Autodesk Inventor part; units mm, degrees
ref_plane "YZ Plane" through (0, 0, 0) normal (1, 0, 0) x (0, 1, 0)
ref_plane "XZ Plane" through (0, 0, 0) normal (0, 1, 0) x (-1, 0, 0)
ref_plane "XY Plane" through (0, 0, 0) normal (0, 0, 1) x (1, 0, 0)
sketch "Skizze1" plane through (0, 0, 0) normal (0, 0, 1) x (1, 0, 0)
  arc A0 (2.449, 9.6955) -> (2.449, -9.6955) centre (0, 0) ccw
  arc A1 (25.4796, -3.8782) -> (25.4796, 3.8782) centre (24.5, 0) ccw
  line L0 (25.4796, 3.8782) -> (2.449, 9.6955)
  line L1 (25.4796, -3.8782) -> (2.449, -9.6955)
  circle A2 centre (0, 0) radius 3.8
  dimension "d0" = 20
  dimension "d1" = 8
  dimension "d2" = 24.5
  dimension "d40" = 7.6
extrude "Extrusion1" add sketch "Skizze1" along normal blind 3.2
sketch "Skizze2" plane through (0, 0, 0) normal (0, 0, -1) x (-1, 0, 0)
  arc A0 (-25.4796, 3.8782) -> (-25.4796, -3.8782) centre (-24.5, 0) ccw
  circle A1 centre (-24.5, 0) radius 4
  point P0 (0, 0)
  point P1 (-25.4796, 3.8782)
extrude "Extrusion2" add sketch "Skizze2" along normal blind 1.2
sketch "Skizze3" plane through (24.5, 0, -1.2) normal (0, 0, -1) x (-1, 0, 0)
  circle A0 centre (0, 0) radius 4
  point P0 (24.5, 0)
hole "Bohrung1" at (24.5, 0, -1.2) direction (0, 0, 1) diameter 6.2 depth 2
sketch "Skizze4" plane through (0, 0, 0) normal (0, 0, -1) x (-1, 0, 0)
  point P0 (0, 0)
  point P1 (0, -7)
  dimension "d14" = 7
hole "Bohrung2" at (0, -7, 0) direction (0, 0, 1) diameter 2.5 end through all
pattern_circular "Runde Anordnung1" count 4 over 360 about axis through (0, 0, 0) along (0, 0, 1) of "Bohrung2"
chamfer "Fasen4" distance 0.2 angle 45 1 edges at (24.5, -3.1, -1.2)
sketch "Skizze5" plane through (24.5, 0, 0.8) normal (0, 0, -1) x (-1, 0, 0)
  circle A0 centre (0, 0) radius 3.1
  point P0 (24.5, 0)
extrude "Extrusion3" cut sketch "Skizze5" against normal blind 0.5
properties part number "Magnet-arm"
Design review of the part built by this model. Coordinates are the model's own, in mm. A direction names the side the tool comes from. Round coordinates to 2 decimals unless told otherwise and drop trailing zeros. Loops run counter-clockwise (first coordinate to the right, second up) from the corner with the lowest first, then second, coordinate; pieces in that order, holes last. Notation, with made-up numbers: (53.5, -16.75) - (108.5, -16.75) arc R33 ccw to (108.5, 12.25) - close; hole circle Ø10 at (39.25, -19). An arc over 180 degrees is marked (long way). One line per item, written item: value. Start each with the question number.
1) Consider section B-B on z = 2.65. Give the boundary of the cut face in (x, y), then the cut area to 3 significant figures.
2) Draft analysis for pull direction Y (two halves, no side actions). For faces 1 (the flat face through (14.126, -6.746, 1.578)), 2 (the cylindrical face through (21.767, 1.463, 0.166)), 3 (the cylindrical face through (-10, 0, 2)), state which applies: +Y half, -Y half, draft (parallel to the pull), parting line (faces both ways), or undercut.
3) Consider section C-C on y = 0. Give the boundary of the cut face in (x, z), then the cut area to 3 significant figures.
4) To check wall thickness, follow L1, parallel to Z at x = 25.5, y = 1.75; L2, parallel to Y at x = 24.5, z = -0.2; L3, parallel to Z at x = 10, y = 6.75. State the ranges of each line that lie inside material, in increasing order. Write a range as from..to.
5) Consider section A-A on x = 0. Give the boundary of the cut face in (y, z), then the cut area to 3 significant figures.
6) Insertion check: pin 1 Ø2 at (x, z) = (-3.5, 2.5) entering from +Y; pin 2 Ø3 at (x, y) = (-7, 0) entering from -Z; pin 3 Ø1.5 at (x, z) = (23.5, 0.5) entering from +Y. Each pin has a flat end and moves straight along its axis. Give the tip position at first contact, or say it passes through.
7) Consider section D-D on x = 7. Give the boundary of the cut face in (y, z).
8) For faces 4 (the cylindrical face through (8.25, -0.05, 1.62)), 5 (the flat face through (25, 0, 1.3)), list the 3-axis set-ups (+Z, -Z, +X, -X, +Y, -Y) from which the entire face can be reached by the end or side of a thin tool; tool diameter is ignored.
Reported:
1. outline: (2.45, -9.7) - (25.48, -3.88) arc R4 ccw to (25.48, 3.88) - (2.45, 9.7) arc R10 ccw (long way) to start; hole circle Ø2.5 at (-7, 0); hole circle Ø7.6 at (0, 0); hole circle Ø2.5 at (0, -7); hole circle Ø2.5 at (0, 7); hole circle Ø2.5 at (7, 0)
1. area: 471 mm^2
2. face 1: -Y half
2. face 2: undercut
2. face 3: parting line
3. outline: (-10, 0) - (-8.25, 0) - (-8.25, 3.2) - (-10, 3.2) - close; (-5.75, 0) - (-3.8, 0) - (-3.8, 3.2) - (-5.75, 3.2) - close; (3.8, 0) - (5.75, 0) - (5.75, 3.2) - (3.8, 3.2) - close; (8.25, 0) - (20.5, 0) - (20.5, -1.2) - (21.2, -1.2) - (21.4, -1) - (21.4, 1.3) - (27.6, 1.3) - (27.6, -1) - (27.8, -1.2) - (28.5, -1.2) - (28.5, 3.2) - (8.25, 3.2) - close
3. area: 76.9 mm^2
4. L1: z = 1.3..3.2
4. L2: y = -4..-3.1, 3.1..4
4. L3: z = 0..3.2
5. outline: (-10, 0) - (-8.25, 0) - (-8.25, 3.2) - (-10, 3.2) - close; (-5.75, 0) - (-3.8, 0) - (-3.8, 3.2) - (-5.75, 3.2) - close; (3.8, 0) - (5.75, 0) - (5.75, 3.2) - (3.8, 3.2) - close; (8.25, 0) - (10, 0) - (10, 3.2) - (8.25, 3.2) - close
5. area: 23.7 mm^2
6. pin 1: stops at y = 9.68
6. pin 2: stops at z = 0
6. pin 3: stops at y = 4.57
7. outline: (-8.55, 0) - (-1.25, 0) - (-1.25, 3.2) - (-8.55, 3.2) - close; (1.25, 0) - (8.55, 0) - (8.55, 3.2) - (1.25, 3.2) - close
8. face 4: +Z, -Z
8. face 5: -Z
